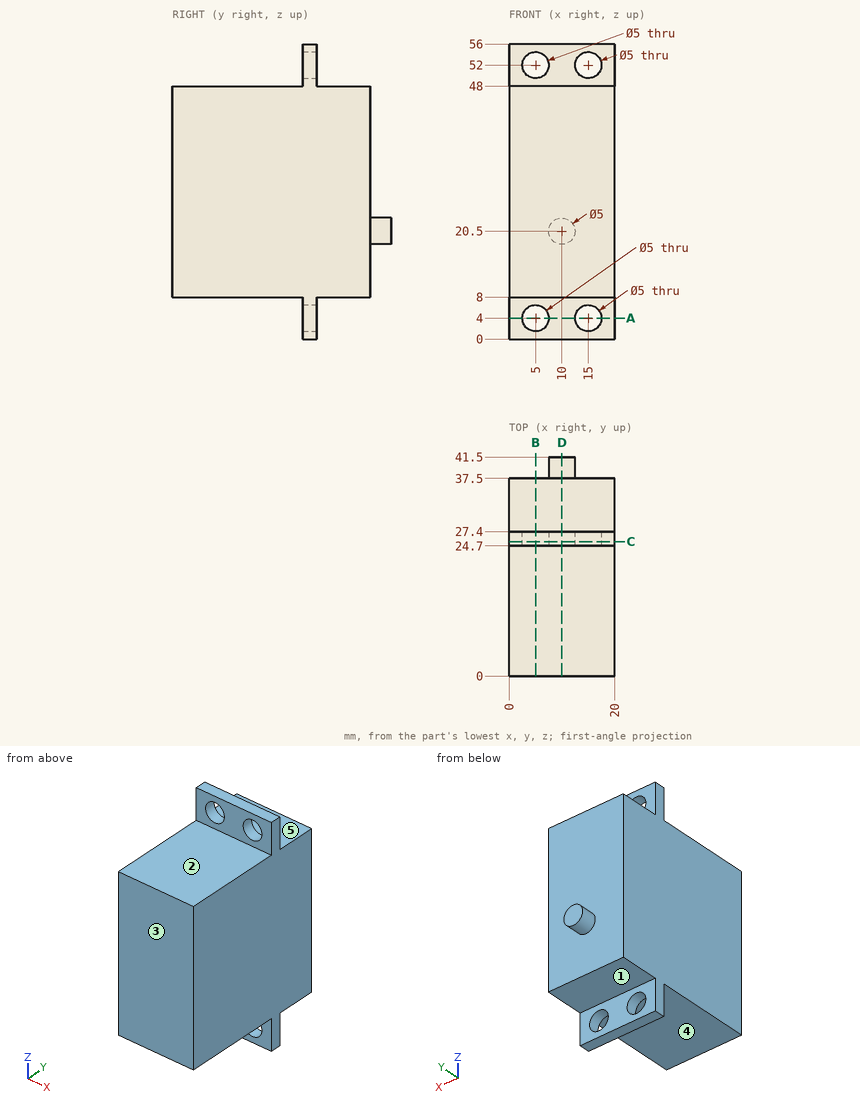
Check sheet for the drawn part. Datum: minimum x, y, z corner. Units: mm. A direction names the side the tool comes from. Round coordinates to 2 decimals unless told otherwise and drop trailing zeros. Write each loop counter-clockwise with the first axis right and the second up, starting at its lowest first coordinate (ties: lowest second). Pieces come first, ordered by that corner, then holes. Notation, with made-up numbers: (56, -13) -> (93, -13) arc R29 cw to (93, 26) -> close; hole circle Ø8 at (48.5, -27.5). An arc over 180 degrees is marked (long way). Put each result on its own line as item: value.
(1) Sectioned sample at A-A (z = 4). Enter the section's corners in (x, y).
Values found:
outline: (0, 24.7) -> (2.5, 24.7) -> (2.5, 27.4) -> (0, 27.4) -> close; (7.5, 24.7) -> (12.5, 24.7) -> (12.5, 27.4) -> (7.5, 27.4) -> close; (17.5, 24.7) -> (20, 24.7) -> (20, 27.4) -> (17.5, 27.4) -> close
(2) Sectioned sample at B-B (x = 5). Enter the section's corners in (y, z), plus the area to 3 significant figures.
Values found:
outline: (0, 8) -> (24.7, 8) -> (24.7, 6.5) -> (27.4, 6.5) -> (27.4, 8) -> (37.5, 8) -> (37.5, 48) -> (27.4, 48) -> (27.4, 49.5) -> (24.7, 49.5) -> (24.7, 48) -> (0, 48) -> close; (24.7, 0) -> (27.4, 0) -> (27.4, 1.5) -> (24.7, 1.5) -> close; (24.7, 54.5) -> (27.4, 54.5) -> (27.4, 56) -> (24.7, 56) -> close
area: 1,520 mm^2
(3) Tool access check on the marked faces 1, 2, 3, 4 and 5. Record the directions out of +Z, -Z, +X, -X, +Y, -Y that give a thin tool (end or side, any length) a straight path to the whole face; none if there is none.
Values found:
face 1: -Z, +X, -X, +Y
face 2: +Z, +X, -X, -Y
face 3: +Z, -Z, +X, -X, -Y
face 4: -Z, +X, -X, -Y
face 5: +Z, +X, -X, +Y
(4) Sectioned sample at C-C (y = 25.5). Enter the section's corners in (x, z).
Values found:
outline: (0, 0) -> (20, 0) -> (20, 56) -> (0, 56) -> close; hole circle Ø5 at (5, 4); hole circle Ø5 at (5, 52); hole circle Ø5 at (15, 4); hole circle Ø5 at (15, 52)
(5) Go/stop test with flat-tipped pins: pin 1 Ø3 at (x, y) = (5.5, 34.5) entering from -Z; pin 2 Ø4 at (x, z) = (11, 5.5) entering from +Y; pin 3 Ø2.5 at (x, z) = (6.5, 52) entering from -Y; pin 4 Ø3 at (x, z) = (5, 52) entering from +Y. Record where each tip stops, or that it passes through.
Values found:
pin 1: stops at z = 8
pin 2: stops at y = 27.4
pin 3: stops at y = 24.7
pin 4: passes through
(6) Material ranges on line 1 (Z direction, x = 15, y = 26.3); line 2 (X direction, y = 25.5, z = 52); line 3 (Z direction, x = 10, y = 23.5), recorded low to high.
Values found:
line 1: z = 0 to 1.5, 6.5 to 49.5, 54.5 to 56
line 2: x = 0 to 2.5, 7.5 to 12.5, 17.5 to 20
line 3: z = 8 to 48
(7) Sectioned sample at D-D (x = 10). Enter the section's corners in (y, z).
Values found:
outline: (0, 8) -> (24.7, 8) -> (24.7, 0) -> (27.4, 0) -> (27.4, 8) -> (37.5, 8) -> (37.5, 18) -> (41.5, 18) -> (41.5, 23) -> (37.5, 23) -> (37.5, 48) -> (27.4, 48) -> (27.4, 56) -> (24.7, 56) -> (24.7, 48) -> (0, 48) -> close
